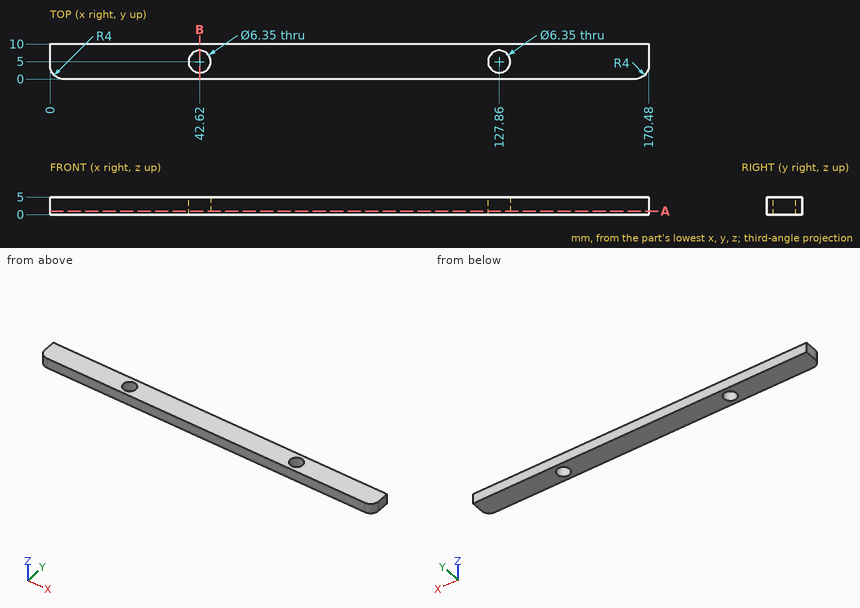
Design review of the part shown in the three views and the two pictorial views. Dimensions are in mm from the part's minimum x, y and z. Give positions to 0.01 mm unless a question says otherwise; leave off trailing zeros. Order: outer loops, then holes, each group sorted by start corner. A loop starts at its lowest first (then second) coordinate and runs counter-clockwise, first axis right, second up. Notation, with made-up numbers: M -23,16.5 L 17,16.5 A27 ccw 17,38.5 Z; hole C 13.25,36.25 d5. An arc over 180 degrees is marked long. Answer in a Markdown table with one row per item. Add a question column.
(1) Consider section B-B on x = 42.62. State the section outline as (y, z) points (3 decimals).
(2) For pin 1 (6 mm diameter, centred on x = 42, y = 4.5, fed in from +Z); pin 2 (4 mm diameter, centred on x = 42.62, y = 5, fed in from -Z), all flat-tipped, find the tip position at first contact; note any pin that passes through.
(3) Consider section A-A on z = 1. State the section outline as (x, y) points (3 decimals), and give its area (3 significant figures).
(4) Wall thickness on probe 1 along Y at (x, z) = (42.62, 3.65) (3 decimals); probe 2 along X at (y, z) = (2.5, 1.45); probe 3 along X at (y, z) = (2.75, 3.8): over which ranges is each line inside the solid? List them lowest first. Write a range as [from, to].
Evaluation:
| question | item | result |
|---|---|---|
| 1 | outline | M 0,0 L 1.825,0 L 1.825,5 L 0,5 Z; M 8.175,0 L 10,0 L 10,5 L 8.175,5 Z |
| 2 | pin 1 | stops at z = 5 |
| 2 | pin 2 | passes through |
| 3 | outline | M 0,4 A4 ccw 4,0 L 166.48,0 A4 ccw 170.48,4 L 170.48,10 L 0,10 Z; hole C 42.62,5 d6.35; hole C 127.86,5 d6.35 |
| 3 | area | 1,630 mm^2 |
| 4 | probe 1 | y = [0, 1.825], [8.175, 10] |
| 4 | probe 2 | x = [0.29, 40.66], [44.58, 125.9], [129.82, 170.19] |
| 4 | probe 3 | x = [0.2, 40.38], [44.86, 125.62], [130.1, 170.28] |
